Could you check a few things on this model? Use its own coordinates, in mm. Face numbers are marked on the shaded views. A direction names the side the tool comes from. Give positions to 0.01 mm unless a question says otherwise; leave off trailing zeros. Write each loop counter-clockwise with the first axis right and the second up, starting at its lowest first coordinate (ties: lowest second). Pieces come first, ordered by that corner, then holes. Notation, with made-up numbers: (46, -7.5) -> (77, -7.5) arc R18 cw to (77, 15.5) -> close; hole circle Ø8 at (-27.75, -6.5). An arc over 180 degrees is marked (long way). One line per question, with ' | ' between items.
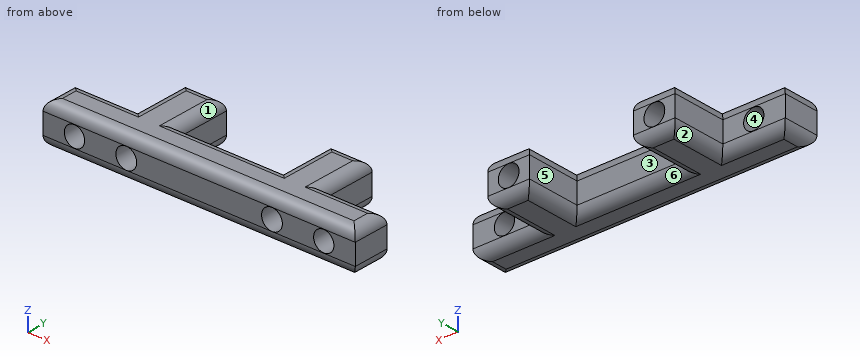
from build123d import *

# Parameters (mm, degrees)
SKETCH1_W           = 60
SKETCH1_H           = 8
BOSS_EXTRUDE1_DEPTH = 7
SKETCH2_W           = 8
SKETCH2_H           = 8
BOSS_EXTRUDE2_DEPTH = 10.5
SKETCH3_R           = 2
CUT_EXTRUDE1_DEPTH  = 35.960692213
SKETCH5_R           = 1.95
CUT_EXTRUDE2_DEPTH  = 35.960692213
FILLET1_R           = 2


with BuildPart() as part:
    # Sketch1 → Boss-Extrude1 (new body)
    with BuildSketch(Plane(origin=(0, 0, 0), x_dir=(1, 0, 0), z_dir=(0, 1, 0))):
        Rectangle(SKETCH1_W, SKETCH1_H)
    extrude(amount=BOSS_EXTRUDE1_DEPTH)

    # Sketch2 → Boss-Extrude2 (add)
    with BuildSketch(Plane(origin=(0, 7, 0), x_dir=(1, 0, 0), z_dir=(0, 1, 0))):
        with Locations((-14, 0)):
            Rectangle(SKETCH2_W, SKETCH2_H)
        with Locations((14, 0)):
            Rectangle(SKETCH2_W, SKETCH2_H)
    extrude(amount=BOSS_EXTRUDE2_DEPTH)

    # Sketch3 → Cut-Extrude1 (cut, through all)
    with BuildSketch(Plane(origin=(0, 17.5, 0), x_dir=(1, 0, 0), z_dir=(0, 1, 0))):
        with Locations(Location((-14, 0, 0), (0, 0, 270))):
            Circle(SKETCH3_R)
        with Locations(Location((14, 0, 0), (0, 0, 270))):
            Circle(SKETCH3_R)
    extrude(amount=-CUT_EXTRUDE1_DEPTH, mode=Mode.SUBTRACT)

    # Sketch5 → Cut-Extrude2 (cut, through all)
    with BuildSketch(Plane.XZ):
        with Locations(Location((-23.95, 0, 0), (0, 0, 270))):
            Circle(SKETCH5_R)
        with Locations(Location((23.95, 0, 0), (0, 0, 270))):
            Circle(SKETCH5_R)
    extrude(amount=-CUT_EXTRUDE2_DEPTH, mode=Mode.SUBTRACT)

    # Fillet1
    fillet1_edges = [part.edges().sort_by_distance(p)[0] for p in [
        (0, 7, -4),
        (-24, 7, -4),
        (0, 7, 4),
        (24, 7, 4),
        (-24, 7, 4),
        (-10, 12.25, 4),
        (-10, 12.25, -4),
        (-18, 12.25, -4),
        (-18, 12.25, 4),
        (-14, 17.5, -4),
        (-14, 17.5, 4),
        (18, 12.25, 4),
        (18, 12.25, -4),
        (10, 12.25, -4),
        (10, 12.25, 4),
        (14, 17.5, -4),
        (14, 17.5, 4),
        (0, 0, 4),
        (0, 0, -4),
        (30, 3.5, 4),
        (-30, 3.5, 4),
        (-30, 3.5, -4),
        (30, 3.5, -4),
        (24, 7, -4),
    ]]
    fillet(fillet1_edges, radius=FILLET1_R - 0.0001)  # a hair under: the kernel refuses the full size


solid = part.part
Q1. If I drill on line 1 along X through (y, z) = (3, 0); line 2 along X through (y, z) = (8.75, 0); line 3 along X through (y, z) = (9, 1.75), over which ranges is the centre line in solid material (lowest first)?
Answer below:
line 1: x = -30 to -25.9, -22 to -16, -12 to 12, 16 to 22, 25.9 to 30 | line 2: x = -18 to -16, -12 to -10, 10 to 12, 16 to 18 | line 3: x = -18 to -14.97, -13.03 to -10, 10 to 13.03, 14.97 to 18
Q2. Imagine slicing it at D-D on y = 3. Please give me the cut outline in (x, z), and give its area (3 significant figures).
Answer below:
outline: (-30, -2) arc R2 ccw to (-28, -4) -> (28, -4) arc R2 ccw to (30, -2) -> (30, 2) arc R2 ccw to (28, 4) -> (-28, 4) arc R2 ccw to (-30, 2) -> close; hole circle Ø3.9 at (-23.95, 0); hole circle Ø4 at (-14, 0); hole circle Ø4 at (14, 0); hole circle Ø3.9 at (23.95, 0) | area: 428 mm^2
Q3. If we mould it in two halves opening along Z, with no side actions, what happens to the marked faces 4, 5 and 6? For each: +Z half, -Z half, draft (parallel to the pull), parting line (faces both ways), or undercut.
Answer below:
face 4: undercut | face 5: draft | face 6: -Z half
Q4. Imagine slicing it at C-C on x = -23.95. Please give me the cut outline in (y, z).
Answer below:
outline: (0, -2) arc R2 ccw to (2, -4) -> (5, -4) arc R2 ccw to (7, -2) -> (7, -1.95) -> (0, -1.95) -> close; (0, 1.95) -> (7, 1.95) -> (7, 2) arc R2 ccw to (5, 4) -> (2, 4) arc R2 ccw to (0, 2) -> close
Q5. Will these pins go through, and if not, where does the flat tip stop? pin 1 (4.5 mm diameter, centred on x = -1, z = 0, fed in from +Y); pin 2 (3 mm diameter, centred on y = 11.5, z = -1, fed in from -X); pin 3 (3 mm diameter, centred on y = 13.5, z = 0.5, fed in from +X); pin 4 (3 mm diameter, centred on x = 23.95, z = 0, fed in from +Y).
Answer below:
pin 1: stops at y = 7 | pin 2: stops at x = -18 | pin 3: stops at x = 18 | pin 4: passes through
Q6. On a 3-axis mill with a long thin cutter (end or side, diameter ignored), from which of +Z, -Z, +X, -X, +Y, -Y can I reach the whole of each face in a straight line? I mean the marked faces 1, 2 and 3. Say none if no direction works.
Answer below:
face 1: +Z, +Y | face 2: -Z, -X, +Y | face 3: +Z, -Z, +Y
Q7. Imagine slicing it at B-B on z = 0. Please give me the cut outline in (x, y).
Answer below:
outline: (-30, 0) -> (-25.9, 0) -> (-25.9, 7) -> (-30, 7) -> close; (-22, 0) -> (-16, 0) -> (-16, 17.5) -> (-18, 17.5) -> (-18, 7) -> (-22, 7) -> close; (-12, 0) -> (12, 0) -> (12, 17.5) -> (10, 17.5) -> (10, 7) -> (-10, 7) -> (-10, 17.5) -> (-12, 17.5) -> close; (16, 0) -> (22, 0) -> (22, 7) -> (18, 7) -> (18, 17.5) -> (16, 17.5) -> close; (25.9, 0) -> (30, 0) -> (30, 7) -> (25.9, 7) -> close
Q8. Imagine slicing it at A-A on y = 11. Please give me the cut outline in (x, z), and give its area (3 significant figures).
Answer below:
outline: (-18, -2) arc R2 ccw to (-16, -4) -> (-12, -4) arc R2 ccw to (-10, -2) -> (-10, 2) arc R2 ccw to (-12, 4) -> (-16, 4) arc R2 ccw to (-18, 2) -> close; (10, -2) arc R2 ccw to (12, -4) -> (16, -4) arc R2 ccw to (18, -2) -> (18, 2) arc R2 ccw to (16, 4) -> (12, 4) arc R2 ccw to (10, 2) -> close; hole circle Ø4 at (-14, 0); hole circle Ø4 at (14, 0) | area: 96.0 mm^2
